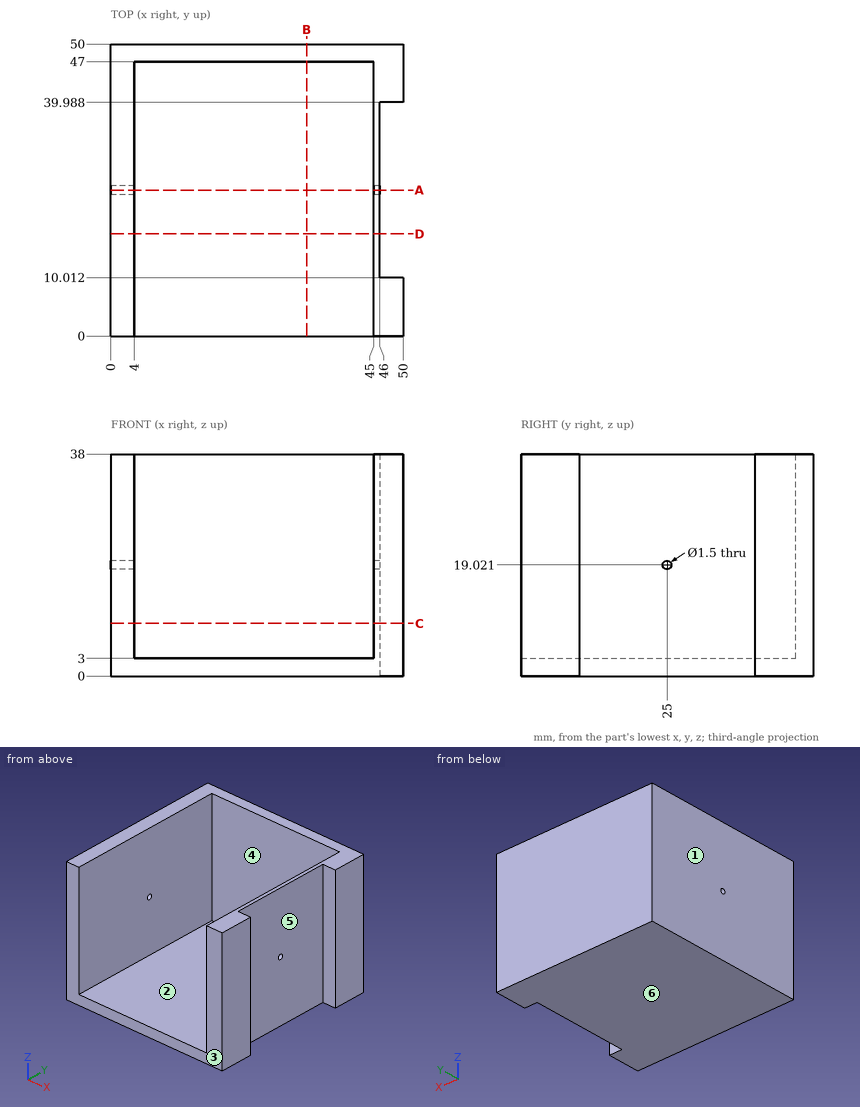
Part print with two shaded views. Sizes in mm from the minimum x, y, z corner. A direction names the side the tool comes from. Round coordinates to 2 decimals unless told otherwise and drop trailing zeros. Order: outer loops, then holes, each group sorted by start corner. A loop starts at its lowest first (then second) coordinate and runs counter-clockwise, first axis right, second up. Notation, with made-up numbers: M 46,-9 L 67,-9 A31 cw 67,19 Z; hole C -38,60 d7. An arc over 180 degrees is marked long. Answer in a Markdown table with one row per item. Add a question column.
Q1. Wall check: L1, parallel to X at y = 19, z = 8; L2, parallel to Z at x = 0.9, y = 25; L3, parallel to X at y = 46, z = 24. Give the ranges that are in metal, low to high. Write a range as from..to.
Q2. Pin check, flat tips, straight feed: pin 1 (1 mm diameter, centred on y = 27, z = 31, fed in from +X); pin 2 (5 mm diameter, centred on x = 35, y = 13.5, fed in from +Z); pin 3 (17.5 mm diameter, centred on x = 21, z = 27.5, fed in from -Y). Stop position of each tip, or through.
Q3. Cut at D-D on y = 17.5. Give the cut face in (x, z).
Q4. Cut at B-B on x = 33.5. Give the cut face in (y, z).
Q5. 3-axis set-ups, long thin cutter, end or side, ignore diameter. For the marked faces 4, 5 and 6: which of +Z, -Z, +X, -X, +Y, -Y reach the whole face in a straight line?
Q6. Cut at A-A on y = 25. Give the cut face in (x, z).
Q7. Cut at C-C on z = 9. Give the cut face in (x, y).
Q8. Mould opens along X. For the marked faces 1, 2 and 3 say: +X half, -X half, draft (parallel to the pull), parting line (faces both ways), or undercut.
Established:
| question | item | result |
|---|---|---|
| 1 | L1 | x = 0..4, 45..46 |
| 1 | L2 | z = 0..18.27, 19.77..38 |
| 1 | L3 | x = 0..4, 45..50 |
| 2 | pin 1 | stops at x = 46 |
| 2 | pin 2 | stops at z = 3 |
| 2 | pin 3 | stops at y = 47 |
| 3 | outline | M 0,0 L 46,0 L 46,38 L 45,38 L 45,3 L 4,3 L 4,38 L 0,38 Z |
| 4 | outline | M 0,0 L 50,0 L 50,38 L 47,38 L 47,3 L 0,3 Z |
| 5 | face 4 | +Z, -Y |
| 5 | face 5 | +Z, -Z, +X |
| 5 | face 6 | -Z, +X, -X, +Y, -Y |
| 6 | outline | M 0,0 L 46,0 L 46,18.27 L 45,18.27 L 45,3 L 4,3 L 4,18.27 L 0,18.27 Z; M 0,19.77 L 4,19.77 L 4,38 L 0,38 Z; M 45,19.77 L 46,19.77 L 46,38 L 45,38 Z |
| 7 | outline | M 0,0 L 4,0 L 4,47 L 45,47 L 45,0 L 50,0 L 50,10.01 L 46,10.01 L 46,39.99 L 50,39.99 L 50,50 L 0,50 Z |
| 8 | face 1 | -X half |
| 8 | face 2 | undercut |
| 8 | face 3 | draft |
